Check sheet for the modelled part. Datum: model origin and axes. Units: mm. Face numbers are marked on the shaded views. A direction names the side the tool comes from. Coordinates: 2 decimals unless noted, no trailing zeros. Order: outer loops, then holes, each group sorted by start corner. A loop starts at its lowest first (then second) coordinate and runs counter-clockwise, first axis right, second up.
from build123d import *

# Parameters (mm, degrees)
EXTRUDE_1_DEPTH     = 4.2
CUT_EXTRUDE_1_REACH = 15.662
SKETCH_3_R          = 1.75
EXTRUDE_2_DEPTH     = 4.2
CHAMFER_1_SIZE      = 1
CUT_EXTRUDE_2_REACH = 15.662
SKETCH_5_W          = 13.93974063
SKETCH_5_H          = 1.4
FILLET_1_R          = 4
CUT_EXTRUDE_3_REACH = 18.927


with BuildPart() as part:
    # 草图1 → 凸台-拉伸1 (new body)
    with BuildSketch(Plane(origin=(0, 0, 0), x_dir=(1, 0, 0), z_dir=(0, 1, 0))):
        with BuildLine():
            Line((0, 5), (7, 5))
            ThreePointArc((7, 5), (12, 0), (7, -5))
            Line((7, -5), (0, -5))
            ThreePointArc((0, -5), (-5, 0), (0, 5))
        make_face()
    extrude(amount=EXTRUDE_1_DEPTH)

    # 草图3 → 切除-拉伸1 (cut, up to next)
    with BuildSketch(Plane.XZ, mode=Mode.PRIVATE) as cut_extrude_1_sk1:
        with Locations(Location((0, 0, 0), (0, 0, 270))):
            Circle(SKETCH_3_R)
    cut_extrude_1_tool1 = extrude(cut_extrude_1_sk1.sketch, amount=-CUT_EXTRUDE_1_REACH, mode=Mode.PRIVATE) & part.part
    add(cut_extrude_1_tool1.solids().sort_by_distance((0, 0, 0))[0], mode=Mode.SUBTRACT)

    # 草图4 → 凸台-拉伸2 (add)
    with BuildSketch(Plane(origin=(0, 4.2, 0), x_dir=(1, 0, 0), z_dir=(0, 1, 0))):
        with BuildLine():
            Line((1, 3), (7, 3))
            ThreePointArc((7, 3), (10, 0), (7, -3))
            Line((7, -3), (1, -3))
            ThreePointArc((1, -3), (-2, 0), (1, 3))
        make_face()
    extrude(amount=EXTRUDE_2_DEPTH)

    # 倒角1
    chamfer_1_edges = [part.edges().sort_by_distance(p)[0] for p in [
        (-2, 8.4, 0),
        (4, 8.4, 3),
        (10, 8.4, 0),
        (4, 8.4, -3),
    ]]
    chamfer(chamfer_1_edges, length=CHAMFER_1_SIZE)

    # 草图5 → 切除-拉伸2 (cut, up to next)
    with BuildSketch(Plane(origin=(0, 4.2, 0), x_dir=(1, 0, 0), z_dir=(0, 1, 0)), mode=Mode.PRIVATE) as cut_extrude_2_sk1:
        with Locations((3.5, -4.3)):
            Rectangle(SKETCH_5_W, SKETCH_5_H)
    cut_extrude_2_tool1 = extrude(cut_extrude_2_sk1.sketch, amount=-CUT_EXTRUDE_2_REACH, mode=Mode.PRIVATE) & part.part
    add(cut_extrude_2_tool1.solids().sort_by_distance((3.5, 4.2, 4.3))[0], mode=Mode.SUBTRACT)

    # 圆角1
    fillet_1_edges = [part.edges().sort_by_distance(p)[0] for p in [
        (-3.469870315, 2.1, 3.6),
        (10.469870315, 2.1, 3.6),
    ]]
    fillet(fillet_1_edges, radius=FILLET_1_R)

    # 草图6 → 切除-拉伸3 (cut, up to next)
    with BuildSketch(Plane.XY.offset(3.6), mode=Mode.PRIVATE) as cut_extrude_3_sk1:
        Polygon((-0.45, 8.4), (-0.1, 7.793782217), (0.25, 8.4), align=None)
    cut_extrude_3_tool1 = extrude(cut_extrude_3_sk1.sketch, amount=-CUT_EXTRUDE_3_REACH, mode=Mode.PRIVATE) & part.part
    # 草图6 → 切除-拉伸3 (cut, up to next)
    with BuildSketch(Plane.XY.offset(3.6), mode=Mode.PRIVATE) as cut_extrude_3_sk2:
        Polygon((1.41, 8.4), (0.71, 8.4), (1.06, 7.793782217), align=None)
    cut_extrude_3_tool2 = extrude(cut_extrude_3_sk2.sketch, amount=-CUT_EXTRUDE_3_REACH, mode=Mode.PRIVATE) & part.part
    # 草图6 → 切除-拉伸3 (cut, up to next)
    with BuildSketch(Plane.XY.offset(3.6), mode=Mode.PRIVATE) as cut_extrude_3_sk3:
        Polygon((2.57, 8.4), (1.87, 8.4), (2.22, 7.793782217), align=None)
    cut_extrude_3_tool3 = extrude(cut_extrude_3_sk3.sketch, amount=-CUT_EXTRUDE_3_REACH, mode=Mode.PRIVATE) & part.part
    # 草图6 → 切除-拉伸3 (cut, up to next)
    with BuildSketch(Plane.XY.offset(3.6), mode=Mode.PRIVATE) as cut_extrude_3_sk4:
        Polygon((3.73, 8.4), (3.03, 8.4), (3.38, 7.793782217), align=None)
    cut_extrude_3_tool4 = extrude(cut_extrude_3_sk4.sketch, amount=-CUT_EXTRUDE_3_REACH, mode=Mode.PRIVATE) & part.part
    # 草图6 → 切除-拉伸3 (cut, up to next)
    with BuildSketch(Plane.XY.offset(3.6), mode=Mode.PRIVATE) as cut_extrude_3_sk5:
        Polygon((4.89, 8.4), (4.19, 8.4), (4.54, 7.793782217), align=None)
    cut_extrude_3_tool5 = extrude(cut_extrude_3_sk5.sketch, amount=-CUT_EXTRUDE_3_REACH, mode=Mode.PRIVATE) & part.part
    # 草图6 → 切除-拉伸3 (cut, up to next)
    with BuildSketch(Plane.XY.offset(3.6), mode=Mode.PRIVATE) as cut_extrude_3_sk6:
        Polygon((6.05, 8.4), (5.35, 8.4), (5.7, 7.793782217), align=None)
    cut_extrude_3_tool6 = extrude(cut_extrude_3_sk6.sketch, amount=-CUT_EXTRUDE_3_REACH, mode=Mode.PRIVATE) & part.part
    # 草图6 → 切除-拉伸3 (cut, up to next)
    with BuildSketch(Plane.XY.offset(3.6), mode=Mode.PRIVATE) as cut_extrude_3_sk7:
        Polygon((7.21, 8.4), (6.51, 8.4), (6.86, 7.793782217), align=None)
    cut_extrude_3_tool7 = extrude(cut_extrude_3_sk7.sketch, amount=-CUT_EXTRUDE_3_REACH, mode=Mode.PRIVATE) & part.part
    # 草图6 → 切除-拉伸3 (cut, up to next)
    with BuildSketch(Plane.XY.offset(3.6), mode=Mode.PRIVATE) as cut_extrude_3_sk8:
        Polygon((8.37, 8.4), (7.67, 8.4), (8.02, 7.793782217), align=None)
    cut_extrude_3_tool8 = extrude(cut_extrude_3_sk8.sketch, amount=-CUT_EXTRUDE_3_REACH, mode=Mode.PRIVATE) & part.part
    # 草图6 → 切除-拉伸3 (cut, up to next)
    with BuildSketch(Plane.XY.offset(3.6), mode=Mode.PRIVATE) as cut_extrude_3_sk9:
        Polygon((9.53, 8.4), (8.83, 8.4), (9.18, 7.793782217), align=None)
    cut_extrude_3_tool9 = extrude(cut_extrude_3_sk9.sketch, amount=-CUT_EXTRUDE_3_REACH, mode=Mode.PRIVATE) & part.part
    add(cut_extrude_3_tool1.solids().sort_by_distance((-0.1, 8.197927, 3.6))[0], mode=Mode.SUBTRACT)
    add(cut_extrude_3_tool2.solids().sort_by_distance((1.06, 8.197927, 3.6))[0], mode=Mode.SUBTRACT)
    add(cut_extrude_3_tool3.solids().sort_by_distance((2.22, 8.197927, 3.6))[0], mode=Mode.SUBTRACT)
    add(cut_extrude_3_tool4.solids().sort_by_distance((3.38, 8.197927, 3.6))[0], mode=Mode.SUBTRACT)
    add(cut_extrude_3_tool5.solids().sort_by_distance((4.54, 8.197927, 3.6))[0], mode=Mode.SUBTRACT)
    add(cut_extrude_3_tool6.solids().sort_by_distance((5.7, 8.197927, 3.6))[0], mode=Mode.SUBTRACT)
    add(cut_extrude_3_tool7.solids().sort_by_distance((6.86, 8.197927, 3.6))[0], mode=Mode.SUBTRACT)
    add(cut_extrude_3_tool8.solids().sort_by_distance((8.02, 8.197927, 3.6))[0], mode=Mode.SUBTRACT)
    add(cut_extrude_3_tool9.solids().sort_by_distance((9.18, 8.197927, 3.6))[0], mode=Mode.SUBTRACT)


solid = part.part
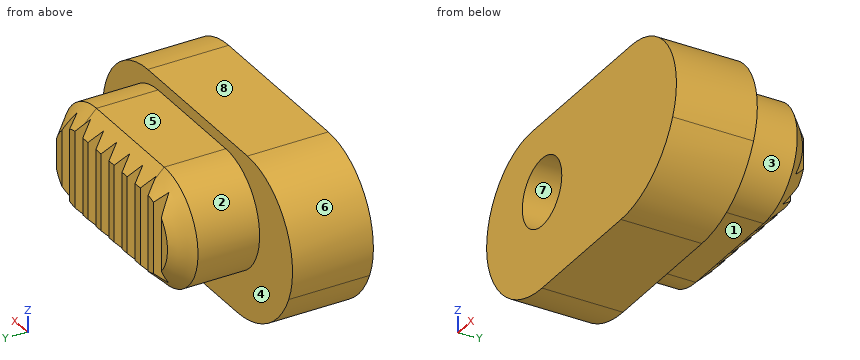
(1) Go/stop test with flat-tipped pins: P1, Ø1.5, axis at x = 5.5, y = 7, coming from the -Z side; P2, Ø2.5, axis at x = 4.5, y = 6, coming from the +Z side; P3, Ø1, axis at x = -0.5, z = -0.5, coming from the -Y side. Record where each tip stops, or that it passes through.
Filled in:
P1: stops at z = -3
P2: stops at z = 3
P3: stops at y = 4.2
(2) Thickness scan on probe 1 along X at (y, z) = (2.5, 0); probe 2 along Y at (x, z) = (-3, 0.25); probe 3 along Z at (x, y) = (5, 7.25). Record the ranges inside material, lowest first.
Filled in:
probe 1: x = -4.9 to -1.75, 1.75 to 11.9
probe 2: y = 0 to 4.2
probe 3: z = -3 to 3
(3) Cross-section at B-B (y = 5.25). Enter the section's corners in (x, z).
Filled in:
outline: (1, -3) - (7, -3) arc R3 ccw to (7, 3) - (1, 3) arc R3 ccw to start
(4) Tool access check on the marked faces 1, 2, 3, 4 and 5. Record the directions out of +Z, -Z, +X, -X, +Y, -Y that give a thin tool (end or side, any length) a straight path to the whole face; none if there is none.
Filled in:
face 1: -Z, +X, -X, +Y
face 2: -X, +Y
face 3: +X, +Y
face 4: +Y
face 5: +Z, +X, -X, +Y
(5) Cross-section at A-A (y = 3.75). Enter the section's corners in (x, z), and give its area (3 significant figures).
Filled in:
outline: (-4.58, -2) arc R5 ccw to (0, -5) - (7, -5) arc R5 ccw to (11.58, -2) arc R4 ccw to (7.92, 3.6) - (-0.92, 3.6) arc R4 ccw to start; hole circle Ø3.5 at (0, 0)
area: 118 mm2
(6) Release check for a two-part mould opening along X. For the marked faces 6, 7 and 8 record: +X half, -X half, draft (parallel to the pull), parting line (faces both ways), or undercut.
Filled in:
face 6: -X half
face 7: undercut
face 8: draft
(7) Cross-section at C-C (x = -3.25). Enter the section's corners in (y, z), and give its area (3 significant figures).
Filled in:
outline: (0, -3.8) - (4.2, -3.8) - (4.2, 2.85) - (0, 2.85) - close
area: 27.9 mm2
